Geometry check sheet. Reference: the model listing, model coordinates, mm. Face numbers are marked on the shaded views. Round coordinates to 2 decimals unless told otherwise and drop trailing zeros. Loops run counter-clockwise (first coordinate to the right, second up) from the corner with the lowest first, then second, coordinate; pieces in that order, holes last. Notation, with made-up numbers: (87, 37) - (124, 37) arc R3 cw to (124, 41) - close; hole circle Ø9 at (59, 54). An arc over 180 degrees is marked (long way). Answer as CSV lines item,"result". Start each with the question number.
1) Thickness scan on line 1 along Z through (x, y) = (0, 14) (3 decimals); line 2 along X through (y, z) = (31.5, -2.5) (3 decimals); line 3 along X through (y, z) = (16, -3) (3 decimals). Record the ranges inside material, lowest first.
2) Cross-section at A-A on y = 9. Record the boundary of the cut face in (x, z) (1 decimal), and give its area (3 significant figures).
3) Depth check by flat-ended pin: P1, Ø10, axis at x = 12.5, y = 7.5, coming from the -Z side (3 decimals); P2, Ø6, axis at x = 9, z = -13.5, coming from the -Y side; P3, Ø1, axis at y = 25, z = 13.5, coming from the +X side; P4, Ø2, axis at x = -12.5, z = -10, coming from the +Y side. Enter the tip coordinate at first touch or a pass-through.
4) Draft check along Z on the marked faces 1, 2, 3 and 4. Enter one of: released by +Z, released by -Z, zero draft, split by the parting line, or undercut.
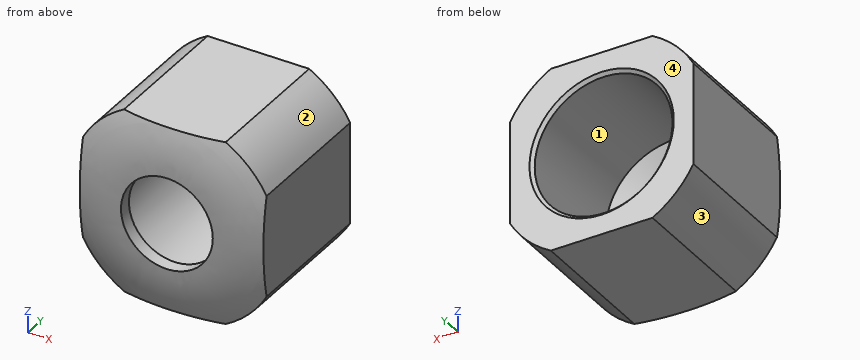
from build123d import *

# Parameters (mm, degrees)
CHAMFER1_SIZE      = 0.79375
CUT_EXTRUDE1_DEPTH = 37.5125001
CIRPATTERN1_COUNT  = 4


with BuildPart() as part:
    # Sketch1 → Revolve1 (revolve)
    with BuildSketch(Plane.XY):
        with BuildLine():
            Line((25.4, 36.5125), (16.66875, 36.5125))
            Line((16.66875, 36.5125), (16.66875, 7.361934691))
            Line((16.66875, 7.361934691), (11.1125, 3.175))
            Line((11.1125, 3.175), (11.1125, 0))
            ThreePointArc((11.1125, 0), (18.430513413, 0.803314642), (25.4, 3.175))
            Line((25.4, 3.175), (25.4, 36.5125))
        make_face()
    revolve(axis=Axis((0, 53.46364703, 0), (0, -1, 0)))

    # Chamfer1
    chamfer1_edges = [part.edges().sort_by_distance(p)[0] for p in [
        (-16.66875, 36.5125, 0),
    ]]
    chamfer(chamfer1_edges, length=CHAMFER1_SIZE)

    # Sketch8 → Cut-Extrude1 (cut, through all)
    with BuildSketch(Plane(origin=(0, 36.5125, 0), x_dir=(1, 0, 0), z_dir=(0, 1, 0))):
        with BuildLine():
            Line((-22.225, 12.296722124), (-22.225, -12.296722124))
            ThreePointArc((-22.225, -12.296722124), (-25.4, 0), (-22.225, 12.296722124))
        make_face()
    cut_extrude1 = extrude(amount=-CUT_EXTRUDE1_DEPTH, mode=Mode.SUBTRACT)

    # CirPattern1: Cut-Extrude1 ×4 about axis
    cirpattern1_axis = Axis((0, 0, 0), (0, 1, 0))
    for i in range(1, CIRPATTERN1_COUNT):
        add(cut_extrude1.rotate(cirpattern1_axis, i * 360 / CIRPATTERN1_COUNT), mode=Mode.SUBTRACT)


solid = part.part
Answer block:
1,line 1,"z = -22.225 to -16.669, 16.669 to 22.225"
1,line 2,"x = -22.225 to -16.48, 16.48 to 22.225"
1,line 3,"x = -22.225 to -16.397, 16.397 to 22.225"
2,outline,"(-22.2, -12.3) arc R25.4 ccw to (-12.3, -22.2) - (12.3, -22.2) arc R25.4 ccw to (22.2, -12.3) - (22.2, 12.3) arc R25.4 ccw to (12.3, 22.2) - (-12.3, 22.2) arc R25.4 ccw to (-22.2, 12.3) - close; hole circle Ø33.3 at (0, 0)"
2,area,"943 mm^2"
3,P1,"stops at z = -22.225"
3,P2,"stops at y = 0.07"
3,P3,"stops at x = 21.82"
3,P4,"stops at y = 36.06"
4,face 1,"undercut"
4,face 2,"released by +Z"
4,face 3,"released by -Z"
4,face 4,"zero draft"
